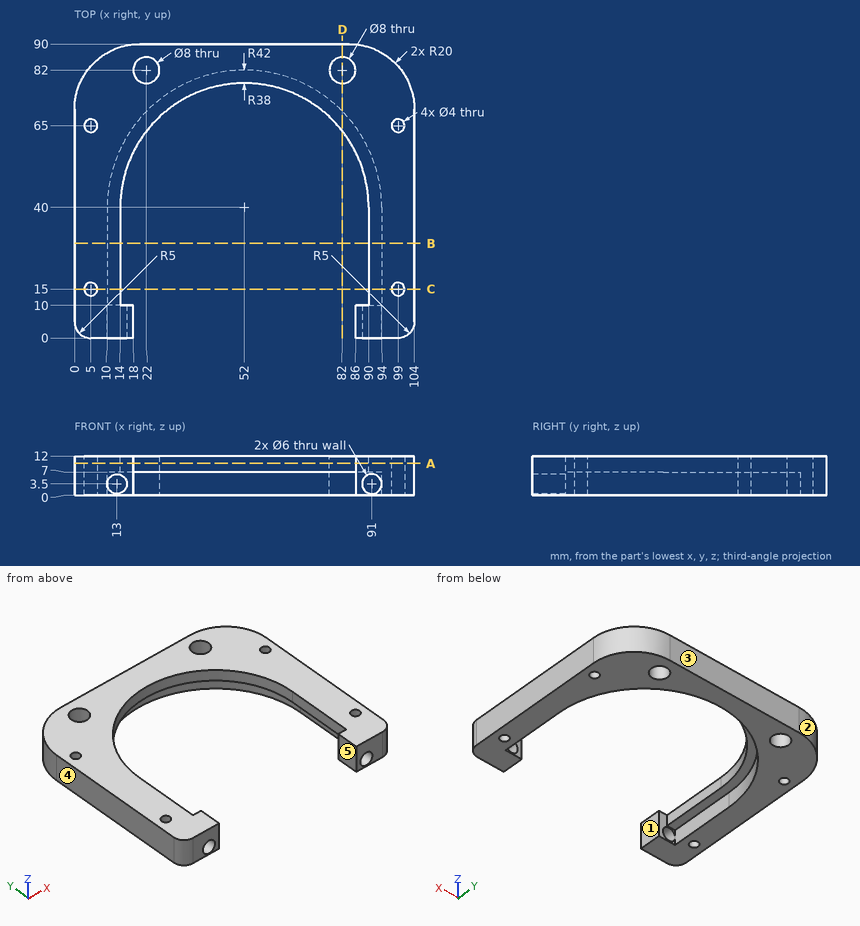
Study the drawing (mm; zero at the part's minimum x, y, z) and answer. A direction names the side the tool comes from. Round coordinates to 2 decimals unless told otherwise and drop trailing zeros. Loops run counter-clockwise (first coordinate to the right, second up) from the corner with the lowest first, then second, coordinate; pieces in that order, holes last.
Q1. Which of the six approach directions +Z, -Z, +X, -X, +Y, -Y give full straight-line access (tool end or side, diameter ignored) to the marked faces 1 and 2?
Q2. Given pin 1 Ø4 at (x, z) = (88.5, 4.5) entering from +Y; pin 2 Ø5 at (x, z) = (13, 3.5) entering from +Y; pin 3 Ø6.5 at (x, z) = (15, 8.5) entering from +Y; pin 4 Ø2.5 at (x, y) = (99, 65) entering from +Z, each flat-ended and moving along its own axis, determine where each tip first touches the part or whether it passes through.
Q3. Section B-B, the plane y = 29 is taken. Determine the outline of the cut face in (x, z).
Q4. Find the intervals of material crossed by line 1 (X direction, y = 83, z = 1.5); line 2 (Z direction, x = 13, y = 2.5); line 3 (X direction, y = 30, z = 5.5), in increasing order.
Q5. For a pull along X with two mould halves and no side action, classify the marked faces 3, 4 and 5 as released by +X, released by -X, zero draft, split by the parting line, or undercut.
Q6. Section C-C, the plane y = 15 is taken. Determine the outline of the cut face in (x, z), then the cut area to 3 significant figures.
Q7. Section D-D, the plane x = 82 is taken. Determine the outline of the cut face in (y, z), then the cut area to 3 significant figures.
Q8. Section A-A, the plane z = 9.75 is taken. Determine the outline of the cut face in (x, y), then the cut area to 3 significant figures.
Completed:
1. face 1: +Z, -Z, -Y
1. face 2: +Z, -Z, -X, +Y
2. pin 1: stops at y = 89.84
2. pin 2: stops at y = 89.49
2. pin 3: stops at y = 89.92
2. pin 4: passes through
3. outline: (0, 0) - (10, 0) - (10, 7) - (14, 7) - (14, 12) - (0, 12) - close; (90, 7) - (94, 7) - (94, 0) - (104, 0) - (104, 12) - (90, 12) - close
4. line 1: x = 4.8 to 18.13, 25.87 to 78.13, 85.87 to 99.2
4. line 2: z = 0 to 0.5, 6.5 to 12
4. line 3: x = 0 to 10, 94 to 104
5. face 3: zero draft
5. face 4: released by -X
5. face 5: undercut
6. outline: (0, 0) - (3, 0) - (3, 12) - (0, 12) - close; (7, 0) - (10, 0) - (10, 7) - (14, 7) - (14, 12) - (7, 12) - close; (90, 7) - (94, 7) - (94, 0) - (97, 0) - (97, 12) - (90, 12) - close; (101, 0) - (104, 0) - (104, 12) - (101, 12) - close
6. area: 184 mm2
7. outline: (63.32, 7) - (69.39, 7) - (69.39, 0) - (78, 0) - (78, 12) - (63.32, 12) - close; (86, 0) - (90, 0) - (90, 12) - (86, 12) - close
7. area: 182 mm2
8. outline: (0, 5) arc R5 ccw to (5, 0) - (18, 0) - (18, 10) - (14, 10) - (14, 40) arc R38 cw to (90, 40) - (90, 10) - (86, 10) - (86, 0) - (99, 0) arc R5 ccw to (104, 5) - (104, 70) arc R20 ccw to (84, 90) - (20, 90) arc R20 ccw to (0, 70) - close; hole circle Ø4 at (5, 15); hole circle Ø4 at (5, 65); hole circle Ø8 at (22, 82); hole circle Ø8 at (82, 82); hole circle Ø4 at (99, 15); hole circle Ø4 at (99, 65)
8. area: 3,800 mm2
